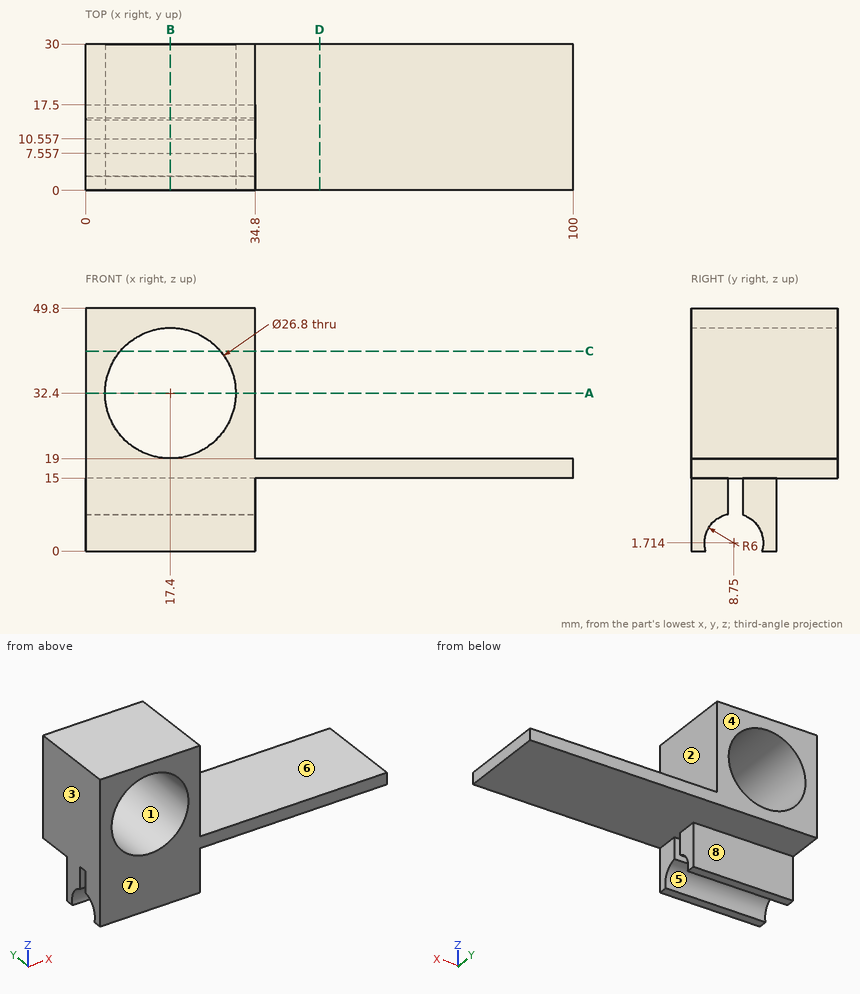
Design review of the part shown in the three views and the two pictorial views. Dimensions are in mm from the part's minimum x, y and z. A direction names the side the tool comes from. Round coordinates to 2 decimals unless told otherwise and drop trailing zeros. Write each loop counter-clockwise with the first axis right and the second up, starting at its lowest first coordinate (ties: lowest second). Pieces come first, ordered by that corner, then holes. Notation, with made-up numbers: M 18.25,6 L 75.25,6 A24 ccw 75.25,24 Z; hole C 48,-27.5 d6. An arc over 180 degrees is marked long. One line per item, written item: value. Start each with the question number.
1. For the marked faces 5, 6, 7 and 8, list the 3-axis set-ups (+Z, -Z, +X, -X, +Y, -Y) from which the entire face can be reached by the end or side of a thin tool; tool diameter is ignored.
2. Take a section at B-B on x = 17.4. State the section outline as (y, z) points.
3. Clearance check with flat-ended pins moving along their axes: P1, Ø8.5, axis at y = 4.5, z = 4.5, coming from the +X side; P2, Ø16, axis at x = 17.4, z = 32.4, coming from the -Y side; P3, Ø12, axis at x = 63, y = 17, coming from the -Z side; P4, Ø9, axis at x = 62, y = 20, coming from the +Z side. State where each tip first meets the part, or that it passes through.
4. To check wall thickness, follow probe 1 along X at (y, z) = (16.5, 32.4); probe 2 along Z at (x, y) = (22, 10.75); probe 3 along Z at (x, y) = (21, 27.25). State the ranges of each line that lie inside material, in increasing order. Write a range as from..to.
5. Draft analysis for pull direction X (two halves, no side actions). For the marked faces 1, 2, 3 and 4, state which applies: pulls with the +X half, pulls with the -X half, needs draft (parallel to the pull), parting line crosses it, or undercut.
6. Take a section at A-A on z = 32.4. State the section outline as (x, y) points, then the cut area to 3 significant figures.
7. Take a section at C-C on z = 41. State the section outline as (x, y) points, then the cut area to 3 significant figures.
8. Take a section at D-D on x = 48. State the section outline as (y, z) points.
Computed:
1. face 5: +X, -X
1. face 6: +Z, +X, +Y, -Y
1. face 7: +Z, -Z, +X, -X, -Y
1. face 8: -Z, +X, -X, +Y
2. outline: M 0,0 L 3,0 A6 cw 7.56,7.59 L 7.56,15 L 10.56,15 L 10.56,7.44 A6 cw 14.5,0 L 17.5,0 L 17.5,15 L 30,15 L 30,19 L 0,19 Z; M 0,45.8 L 30,45.8 L 30,49.8 L 0,49.8 Z
3. P1: stops at x = 34.8
3. P2: passes through
3. P3: stops at z = 15
3. P4: stops at z = 19
4. probe 1: x = 0..4, 30.8..34.8
4. probe 2: z = 7.37..19.81, 44.99..49.8
4. probe 3: z = 15..19.49, 45.31..49.8
5. face 1: undercut
5. face 2: pulls with the +X half
5. face 3: pulls with the -X half
5. face 4: needs draft
6. outline: M 0,0 L 4,0 L 4,30 L 0,30 Z; M 30.8,0 L 34.8,0 L 34.8,30 L 30.8,30 Z
6. area: 240 mm²
7. outline: M 0,0 L 7.12,0 L 7.12,30 L 0,30 Z; M 27.68,0 L 34.8,0 L 34.8,30 L 27.68,30 Z
7. area: 427 mm²
8. outline: M 0,15 L 30,15 L 30,19 L 0,19 Z
